For this review, take the finished solid that the model builds, in its own axes (mm). Give positions to 0.01 mm unless a question says otherwise; leave off trailing zeros. Loops run counter-clockwise (first coordinate to the right, second up) from the corner with the lowest first, then second, coordinate; pieces in that order, holes last. Notation, with made-up numbers: (-21, 3) - (1, 3) arc R12 cw to (1, 13) - close; hole circle Ø5 at (77.5, 49.25). An arc over 180 degrees is marked (long way). Put each result on its own line as item: value.
from build123d import *

# Parameters (mm, degrees)
SKETCH1_R           = 2.25
BOSS_EXTRUDE1_DEPTH = 1


with BuildPart() as part:
    # Sketch1 → Boss-Extrude1 (new body)
    with BuildSketch(Plane.XY):
        with BuildLine():
            Line((20, 42.5), (20, 47.75))
            ThreePointArc((20, 47.75), (19.414213562, 49.164213562), (18, 49.75))
            Line((18, 49.75), (-10, 49.75))
            Line((-10, 49.75), (-10, -9.25))
            Line((-10, -9.25), (18, -9.25))
            ThreePointArc((18, -9.25), (19.414213562, -8.664213562), (20, -7.25))
            Line((20, -7.25), (20, -2))
            ThreePointArc((20, -2), (19.414213562, -0.585786438), (18, 0))
            Line((18, 0), (0, 0))
            Line((0, 0), (0, 40.5))
            Line((0, 40.5), (18, 40.5))
            ThreePointArc((18, 40.5), (19.414213562, 41.085786438), (20, 42.5))
        make_face()
        with Locations((5.25, 44.75)):
            Circle(SKETCH1_R, mode=Mode.SUBTRACT)
        with Locations((14.75, 44.75)):
            Circle(SKETCH1_R, mode=Mode.SUBTRACT)
        with Locations((14.75, -4.25)):
            Circle(SKETCH1_R, mode=Mode.SUBTRACT)
        with Locations((5.25, -4.25)):
            Circle(SKETCH1_R, mode=Mode.SUBTRACT)
    extrude(amount=BOSS_EXTRUDE1_DEPTH)


solid = part.part
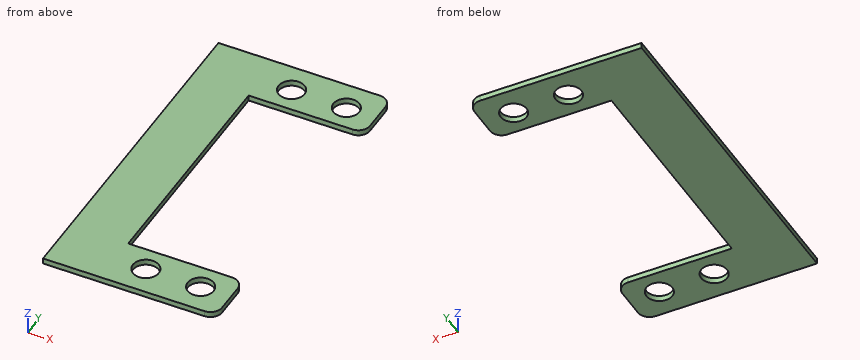
1) Take a section at A-A on y = 44.75. State the section outline as (x, z) points, and give its area (3 significant figures).
Geometry check:
outline: (-10, 0) - (3, 0) - (3, 1) - (-10, 1) - close; (7.5, 0) - (12.5, 0) - (12.5, 1) - (7.5, 1) - close; (17, 0) - (20, 0) - (20, 1) - (17, 1) - close
area: 21.0 mm²
2) Insertion check: pin 1 Ø4 at (x, y) = (14.75, 44.75) entering from +Z; pin 2 Ø0.5 at (y, z) = (11, 0.5) entering from +X. Each pin has a flat end and moves straight along its axis. Give the tip position at first contact, or say it passes through.
Geometry check:
pin 1: passes through
pin 2: stops at x = 0
3) Take a section at D-D on x = 14.75. State the section outline as (y, z) points, and give its area (3 significant figures).
Geometry check:
outline: (-9.25, 0) - (-6.5, 0) - (-6.5, 1) - (-9.25, 1) - close; (-2, 0) - (0, 0) - (0, 1) - (-2, 1) - close; (40.5, 0) - (42.5, 0) - (42.5, 1) - (40.5, 1) - close; (47, 0) - (49.75, 0) - (49.75, 1) - (47, 1) - close
area: 9.50 mm²
4) Take a section at B-B on x = 2.25. State the section outline as (y, z) points, and give its area (3 significant figures).
Geometry check:
outline: (-9.25, 0) - (0, 0) - (0, 1) - (-9.25, 1) - close; (40.5, 0) - (49.75, 0) - (49.75, 1) - (40.5, 1) - close
area: 18.5 mm²
5) Take a section at C-C on z = 0.5. State the section outline as (x, y) points, and give its area (3 significant figures).
Geometry check:
outline: (-10, -9.25) - (18, -9.25) arc R2 ccw to (20, -7.25) - (20, -2) arc R2 ccw to (18, 0) - (0, 0) - (0, 40.5) - (18, 40.5) arc R2 ccw to (20, 42.5) - (20, 47.75) arc R2 ccw to (18, 49.75) - (-10, 49.75) - close; hole circle Ø4.5 at (5.25, -4.25); hole circle Ø4.5 at (5.25, 44.75); hole circle Ø4.5 at (14.75, -4.25); hole circle Ø4.5 at (14.75, 44.75)
area: 893 mm²
6) Wall thickness on line 1 (Y direction, x = 5.25, z = 0.7); line 2 (Y direction, x = 8.25, z = 0.3); line 3 (Y direction, x = 6.5, z = 0.25): over which ranges is each line inside the solid? List them lowest first.
Geometry check:
line 1: y = -9.25 to -6.5, -2 to 0, 40.5 to 42.5, 47 to 49.75
line 2: y = -9.25 to 0, 40.5 to 49.75
line 3: y = -9.25 to -6.12, -2.38 to 0, 40.5 to 42.88, 46.62 to 49.75
